Solid Edge part; units mm, degrees
sketch "Sketch1" plane through (0, 0, 0) normal (0, -1, 0) x (1, 0, 0)
  circle A0 centre (0, 0) radius 1.5
extrude "Protrusion1" add sketch "Sketch1" along normal blind 8
sketch "Sketch2" plane through (0, -8, 0) normal (0, -1, 0) x (-1, 0, 0)
  circle A0 centre (-0.4743, 0) radius 3
extrude "ExtrudedProtrusion_2" add sketch "Sketch2" along normal blind 3
sketch "Sketch3" plane through (0, -11, 0) normal (0, -1, 0) x (1, 0, 0)
  line L0 (1.7243, -0.7217) -> (1.7243, 0.7217)
  line L1 (1.7243, 0.7217) -> (0.4743, 1.4434)
  line L2 (0.4743, 1.4434) -> (-0.7757, 0.7217)
  line L3 (-0.7757, 0.7217) -> (-0.7757, -0.7217)
  line L4 (-0.7757, -0.7217) -> (0.4743, -1.4434)
  line L5 (0.4743, -1.4434) -> (1.7243, -0.7217)
extrude "ExtrudedCutout_2" cut sketch "Sketch3" against normal blind 1.3
properties material "Nylon, general purpose"
Read the model definition and answer for the solid it produces. Units are mm, in the model's axes. A direction names the side the tool comes from. Give positions to 0.01 mm unless a question says otherwise; leave off trailing zeros. Write each loop counter-clockwise with the first axis right and the second up, starting at its lowest first coordinate (ties: lowest second). Pieces come first, ordered by that corner, then holes. Notation, with made-up numbers: (-32, -24) - (-6, -24) arc R16 ccw to (-6, -16) - close; hole circle Ø9 at (23, 45.25). An arc over 180 degrees is marked (long way). Return JSON: item names as keys, results as strings.
Q1. A cutting plane is placed at B-B, the plane x = 0.7. Determine the outline of the cut face in (y, z).
Reply:
{"outline": "(-11, -2.99) - (-8, -2.99) - (-8, -1.33) - (0, -1.33) - (0, 1.33) - (-8, 1.33) - (-8, 2.99) - (-11, 2.99) - (-11, 1.31) - (-9.7, 1.31) - (-9.7, -1.31) - (-11, -1.31) - close"}
Q2. Consider line 1 along Y through (x, z) = (-1.3, -1.3); line 2 along Y through (x, z) = (0.55, 1.25); line 3 along Z through (x, y) = (-0.4, -2.5). Determine where each line is inside the solid, lowest interval first. Write a range as [from, to].
Reply:
{"line 1": "[-11, -8]", "line 2": "[-9.7, 0]", "line 3": "[-1.45, 1.45]"}
Q3. For faces 4 (the face through (-1, -11, 0)), 5 (the face through (-1.5, -3.94, -0.07)), 6 (the face through (-0.159, -10.359, -1.077)), determine the directions among +Z, -Z, +X, -X, +Y, -Y from which every point of the face is accessible in a straight line to the end or side of a thin tool.
Reply:
{"face 4": "+Z, -Z, +X, -X, -Y", "face 5": "+Y", "face 6": "-Y"}
Q4. A cutting plane is placed at A-A, the plane z = 0. Determine the outline of the cut face in (x, y), and give its area (4 significant figures).
Reply:
{"outline": "(-2.53, -11) - (-0.78, -11) - (-0.78, -9.7) - (1.72, -9.7) - (1.72, -11) - (3.47, -11) - (3.47, -8) - (1.5, -8) - (1.5, 0) - (-1.5, 0) - (-1.5, -8) - (-2.53, -8) - close", "area": "38.75 mm²"}
Q5. A cutting plane is placed at C-C, the plane y = -4.5. Determine the outline of the cut face in (x, z).
Reply:
{"outline": "circle Ø3 at (0, 0)"}
Q6. A cutting plane is placed at D-D, the plane x = -2.1. Determine the outline of the cut face in (y, z), and give its area (3 significant figures).
Reply:
{"outline": "(-11, -1.54) - (-8, -1.54) - (-8, 1.54) - (-11, 1.54) - close", "area": "9.24 mm²"}
Q7. For a pull along X with two mould halves and no side action, classify faces 1 (the face through (2, -8, 0)), 2 (the face through (1.108, -10.359, 1.077)), 3 (the face through (2.85, -9.48, -1.83)) as released by +X, released by -X, zero draft, split by the parting line, or undercut.
Reply:
{"face 1": "zero draft", "face 2": "undercut", "face 3": "split by the parting line"}
Q8. Given P1, Ø2, axis at y = -3, z = 1.5, coming from the +X side; P2, Ø3, axis at y = -1.5, z = 0.5, coming from the -X side; P3, Ø1.4, axis at y = -10, z = 0.5, coming from the -X side, each flat-ended and moving along its own axis, determine where each tip first touches the part or whether it passes through.
Reply:
{"P1": "x = 1.41", "P2": "x = -1.5", "P3": "x = -2.53"}
